Input: part model. Units: mm. Frame: model coordinates. Coordinates: 2 decimals unless noted, no trailing zeros. Write each loop counter-clockwise with the first axis right and the second up, starting at its lowest first coordinate (ties: lowest second). Pieces come first, ordered by that corner, then holes. Notation, with made-up numbers: (23.5, -27.75) - (71.5, -27.75) arc R33 ccw to (71.5, 1.25) - close; hole circle Ø8 at (44.5, -5.75). An arc over 180 degrees is marked (long way). Use CSV: the item, a comma, the result in double quotes.
```python
from build123d import *

# Parameters (mm, degrees)
SKIZZE1_R                       = 2.5
SKIZZE1_R_2                     = 5
AUFSATZ_LINEAR_AUSTRAGEN1_DEPTH = 7.5


with BuildPart() as part:
    # Skizze1 → Aufsatz-Linear austragen1 (new, symmetric)
    with BuildSketch(Plane.XY):
        with BuildLine():
            Line((-204.917893678, -153), (-375, -153))
            Line((-375, -153), (-375, 97))
            Line((-375, 97), (-107.923048454, 97))
            ThreePointArc((-107.923048454, 97), (-104.817219913, 96.591109915), (-101.923048454, 95.392304845))
            Line((-101.923048454, 95.392304845), (14, 28.464101615))
            ThreePointArc((14, 28.464101615), (18.392304845, 24.07179677), (20, 18.07179677))
            Line((20, 18.07179677), (20, 15))
            Line((20, 15), (20, -18.07179677))
            ThreePointArc((20, -18.07179677), (18.392304845, -24.07179677), (14, -28.464101615))
            Line((14, -28.464101615), (-198.917893678, -151.392304845))
            ThreePointArc((-198.917893678, -151.392304845), (-201.812065137, -152.591109915), (-204.917893678, -153))
        make_face()
        with Locations((-270, -16)):
            Circle(SKIZZE1_R, mode=Mode.SUBTRACT)
        with Locations((-360, 7)):
            Circle(SKIZZE1_R_2, mode=Mode.SUBTRACT)
        with Locations((-360, -133)):
            Circle(SKIZZE1_R_2, mode=Mode.SUBTRACT)
        with Locations((-90, -16)):
            Circle(SKIZZE1_R, mode=Mode.SUBTRACT)
        with Locations((10, 16)):
            Circle(SKIZZE1_R, mode=Mode.SUBTRACT)
    extrude(amount=AUFSATZ_LINEAR_AUSTRAGEN1_DEPTH, both=True)


solid = part.part
```
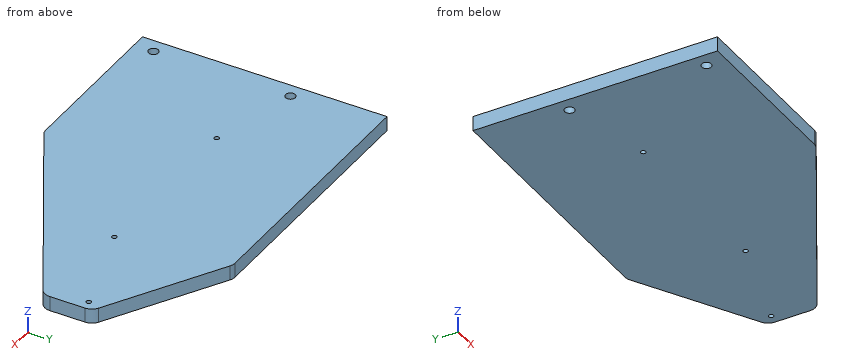
(1) Ray query, probe 1 along Y at (x, z) = (-360, 2); probe 2 along X at (y, z) = (-15.5, 3.75); probe 3 along Y at (x, z) = (-270, -2.5). Return the intervals inside material, ascending. Write a range as from..to.
Check values:
probe 1,"-153..-138, -128..2, 12..97"
probe 2,"-375..-272.45, -267.55..-92.45, -87.55..20"
probe 3,"-153..-18.5, -13.5..97"
(2) Cut plane A-A on y = 7. Return loops of the section in (x, z), and give its area (4 significant figures).
Check values:
outline,"(-375, -7.5) - (-365, -7.5) - (-365, 7.5) - (-375, 7.5) - close; (-355, -7.5) - (20, -7.5) - (20, 7.5) - (-355, 7.5) - close"
area,"5,775 mm^2"
(3) Cut plane B-B on z = -4.5. Return loops of the section in (x, y).
Check values:
outline,"(-375, -153) - (-204.92, -153) arc R12 ccw to (-198.92, -151.39) - (14, -28.46) arc R12 ccw to (20, -18.07) - (20, 18.07) arc R12 ccw to (14, 28.46) - (-101.92, 95.39) arc R12 ccw to (-107.92, 97) - (-375, 97) - close; hole circle Ø10 at (-360, -133); hole circle Ø10 at (-360, 7); hole circle Ø5 at (-270, -16); hole circle Ø5 at (-90, -16); hole circle Ø5 at (10, 16)"
(4) Cut plane D-D on x = -155. Return loops of the section in (y, z), and give its area (3 significant figures).
Check values:
outline,"(-126.04, -7.5) - (97, -7.5) - (97, 7.5) - (-126.04, 7.5) - close"
area,"3,350 mm^2"
(5) Cut plane C-C on y = -133. Return loops of the section in (x, z), and give its area (3 significant figures).
Check values:
outline,"(-375, -7.5) - (-365, -7.5) - (-365, 7.5) - (-375, 7.5) - close; (-355, -7.5) - (-167.06, -7.5) - (-167.06, 7.5) - (-355, 7.5) - close"
area,"2,970 mm^2"
(6) Pin query (flat end, axial travel): pin 1 Ø8 at (x, y) = (10, 16) entering from +Z; pin 2 Ø8 at (x, z) = (-59, -4.5) entering from +Y. Return the tip coordinate at first contact, or that it passes through.
Check values:
pin 1,"z = 7.5"
pin 2,"y = 72.92"
